Verification items for the finished model (mm, model axes). A direction names the side the tool comes from. Give positions to 0.01 mm unless a question says otherwise; leave off trailing zeros. Loops run counter-clockwise (first coordinate to the right, second up) from the corner with the lowest first, then second, coordinate; pieces in that order, holes last. Notation, with made-up numbers: M 72.25,65.5 L 98.25,65.5 A24 cw 98.25,89.5 Z; hole C 42,-10.75 d9. An arc over 180 degrees is marked long. Use a Markdown table: item, result.
from build123d import *

# Parameters (mm, degrees)
SKETCH2_R           = 5
BOSS_EXTRUDE1_DEPTH = 50
SKETCH3_R           = 3
BOSS_EXTRUDE2_DEPTH = 10
BOSS_EXTRUDE2_TAPER = 1
SKETCH5_R           = 3
BOSS_EXTRUDE3_DEPTH = 10


with BuildPart() as part:
    # Sketch2 → Boss-Extrude1 (new body)
    with BuildSketch(Plane.XY):
        Circle(SKETCH2_R)
    extrude(amount=BOSS_EXTRUDE1_DEPTH)

    # Sketch3 → Boss-Extrude2 (add)
    with BuildSketch(Plane(origin=(0, 0, 0), x_dir=(-1, 0, 0), z_dir=(0, 0, -1))):
        Circle(SKETCH3_R)
    extrude(amount=BOSS_EXTRUDE2_DEPTH, taper=BOSS_EXTRUDE2_TAPER)

    # Sketch4 → Revolve1 (revolve)
    with BuildSketch(Plane(origin=(0, 0, -10), x_dir=(-1, 0, 0), z_dir=(0, 0, -1))):
        with BuildLine():
            Line((0, 2.825449351), (0, -2.825449351))
            ThreePointArc((0, -2.825449351), (-2.825449351, 0), (0, 2.825449351))
        make_face()
    revolve(axis=Axis((0, 2.825449351, -10), (0, -1, 0)))

    # Sketch5 → Boss-Extrude3 (add)
    with BuildSketch(Plane.XY.offset(50)):
        Circle(SKETCH5_R)
    extrude(amount=BOSS_EXTRUDE3_DEPTH)

    # Sketch6 → Revolve2 (revolve)
    with BuildSketch(Plane.XY.offset(60)):
        with BuildLine():
            Line((0, 3), (0, -3))
            ThreePointArc((0, -3), (-3, 0), (0, 3))
        make_face()
    revolve(axis=Axis((0, 3, 60), (0, -1, 0)))


solid = part.part
(1) Set-up check for faces 1 (the cylindrical face through (-1.08, -4.88, 24.65)), 2 (the flat face through (-0.1, -3.3, 0)), 3 (the flat face through (-0.1, -3.3, 50)): record each of +Z, -Z, +X, -X, +Y, -Y from which the full face is reachable in a straight line by a thin tool's end or side.
Results below:
| item | result |
|---|---|
| face 1 | +Z, -Z |
| face 2 | -Z |
| face 3 | +Z |
(2) Cross-section at B-B on z = 35. Record the cut outline in (x, y).
Results below:
| item | result |
|---|---|
| outline | C 0,0 d10 |
(3) Cross-section at A-A on x = -4. Record the cut outline in (y, z).
Results below:
| item | result |
|---|---|
| outline | M -3,0 L 3,0 L 3,50 L -3,50 Z |
(4) Gauge pin test, flat ends, axial feed: P1, Ø3, axis at y = -3, z = 42, coming from the +X side; P2, Ø2, axis at x = 2.5, y = -2.5, coming from the -Z side; P3, Ø1, axis at x = -3, z = 5.5, coming from the -Y side. Record the tip position at first contact, or that the pin passes through.
Results below:
| item | result |
|---|---|
| P1 | x = 4.77 |
| P2 | z = -11.25 |
| P3 | y = -4.33 |
(5) Material ranges on line 1 (Z direction, x = -0.75, y = -3); line 2 (X direction, y = 4, z = 47.5); line 3 (Y direction, x = -0.25, z = 28), recorded low to high.
Results below:
| item | result |
|---|---|
| line 1 | 0 to 50 |
| line 2 | -3 to 3 |
| line 3 | -4.99 to 4.99 |
